Input: part model. Units: mm. Frame: model coordinates. Face numbers are marked on the shaded views. A direction names the side the tool comes from. Round coordinates to 2 decimals unless told otherwise and drop trailing zeros. Loops run counter-clockwise (first coordinate to the right, second up) from the corner with the lowest first, then second, coordinate; pieces in that order, holes last.
1) Section D-D, the plane x = 56.65. Return loops of the section in (y, z).
2) Section B-B, the plane x = 41.15. Return loops of the section in (y, z).
3) Section C-C, the plane z = 12. State how many separate pieces and enclosed holes the cut face has, and give its area (4 significant figures).
4) Access query for the marked faces 5, 6, 7, 8 and 9. Directions: +Z, -Z, +X, -X, +Y, -Y. A direction counts if a zero-diameter tool reaches every point of the face in a straight line with its end or side. Return the directions, or none.
5) Draft query along X for the marked faces 1, 2, 3 and 4. Return one class per face: pulls with the +X half, pulls with the -X half, needs draft (parallel to the pull), parting line crosses it, or undercut.
6) First-contact query: pin 1 (7.5 mm diameter, centred on x = 56.65, y = 14.35, fed in from +Z); pin 2 (4 mm diameter, centred on x = 25.65, y = 44.5, fed in from +Z); pin 3 (4 mm diameter, centred on y = 41, z = 7, fed in from -X); pin 4 (4.5 mm diameter, centred on y = 37, z = 7.5, fed in from +X). Flat tips, straight axial feed; report the tip coordinate or a pass-through.
7) Ray query, line 1 along Y through (x, z) = (56.65, 2.5); line 2 along X through (y, z) = (10, 3.8); line 3 along Y through (x, z) = (56.65, 12.85). Return the intervals inside material, ascending.
8) Section A-A, the plane y = 10. Return loops of the section in (x, z), and give its area (3 significant figures).
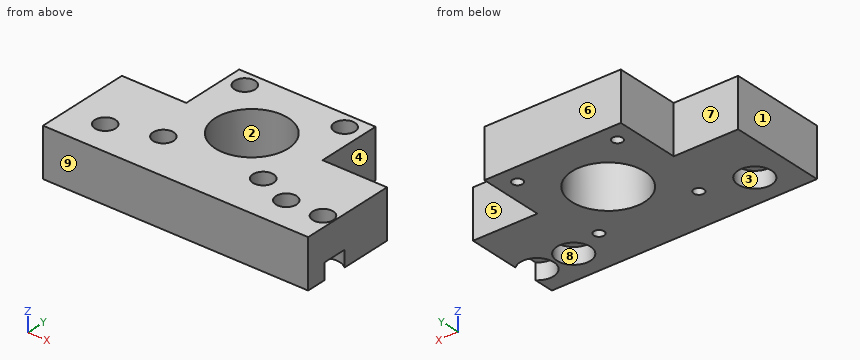
from build123d import *

# Parameters (mm, degrees)
SKETCH_R        = 11.3
SKETCH_R_2      = 1.6
SKETCH_R_3      = 3.2
PAD_DEPTH       = 15
SKETCH001_R     = 3.2
POCKET_DEPTH    = 4
SKETCH002_R     = 5.2
POCKET001_DEPTH = 5


with BuildPart() as part:
    # Sketch → Pad (new body)
    with BuildSketch(Plane.XY):
        Polygon((20, 30), (20, 50.15), (62.3, 50.15), (62.3, 30), (82.3, 30), (82.3, 0), (0, 0), (0, 30), align=None)
        with Locations((41.15, 29)):
            Circle(SKETCH_R, mode=Mode.SUBTRACT)
        with Locations((25.65, 44.5)):
            Circle(SKETCH_R_2, mode=Mode.SUBTRACT)
        with Locations((25.65, 13.5)):
            Circle(SKETCH_R_2, mode=Mode.SUBTRACT)
        with Locations((56.65, 44.5)):
            Circle(SKETCH_R_2, mode=Mode.SUBTRACT)
        with Locations((56.65, 13.5)):
            Circle(SKETCH_R_2, mode=Mode.SUBTRACT)
        with Locations((11.15, 10)):
            Circle(SKETCH_R_3, mode=Mode.SUBTRACT)
        with Locations((67.35, 10)):
            Circle(SKETCH_R_3, mode=Mode.SUBTRACT)
        with Locations((78.75, 10)):
            Circle(SKETCH_R_3, mode=Mode.SUBTRACT)
    extrude(amount=PAD_DEPTH)

    # Sketch001 (on Face18 of Pad) → Pocket (cut)
    with BuildSketch(Plane.XY.offset(15)):
        with Locations((25.65, 45.35)):
            Circle(SKETCH001_R)
        with Locations((56.65, 45.35)):
            Circle(SKETCH001_R)
        with Locations((56.65, 14.35)):
            Circle(SKETCH001_R)
        with Locations((25.65, 14.35)):
            Circle(SKETCH001_R)
    extrude(amount=-POCKET_DEPTH, mode=Mode.SUBTRACT)

    # Sketch002 (on Face4 of Pocket) → Pocket001 (cut)
    with BuildSketch(Plane(origin=(0, 0, 0), x_dir=(1, 0, 0), z_dir=(0, 0, -1))):
        with Locations((11.15, -10)):
            Circle(SKETCH002_R)
        with Locations((67.35, -10)):
            Circle(SKETCH002_R)
        with Locations((78.75, -10)):
            Circle(SKETCH002_R)
    extrude(amount=-POCKET001_DEPTH, mode=Mode.SUBTRACT)


solid = part.part
Final values:
1. outline: (0, 0) - (11.9, 0) - (11.9, 11) - (11.15, 11) - (11.15, 15) - (0, 15) - close; (15.1, 0) - (42.9, 0) - (42.9, 11) - (42.15, 11) - (42.15, 15) - (17.55, 15) - (17.55, 11) - (15.1, 11) - close; (46.1, 0) - (50.15, 0) - (50.15, 15) - (48.55, 15) - (48.55, 11) - (46.1, 11) - close
2. outline: (0, 0) - (17.7, 0) - (17.7, 15) - (0, 15) - close; (40.3, 0) - (50.15, 0) - (50.15, 15) - (40.3, 15) - close
3. separate pieces: 1
3. enclosed holes: 8
3. area: 2,695 mm2
4. face 5: +Z, -Z, +X, +Y
4. face 6: +Z, -Z, +X, -X, +Y
4. face 7: +Z, -Z, -X, +Y
4. face 8: -Z
4. face 9: +Z, -Z, +X, -X, -Y
5. face 1: pulls with the -X half
5. face 2: undercut
5. face 3: undercut
5. face 4: pulls with the +X half
6. pin 1: stops at z = 15
6. pin 2: stops at z = 11
6. pin 3: stops at x = 20
6. pin 4: stops at x = 62.3
7. line 1: y = 0 to 11.9, 15.1 to 42.9, 46.1 to 50.15
7. line 2: x = 0 to 5.95, 16.35 to 62.15, 72.55 to 73.55
7. line 3: y = 0 to 11.15, 17.55 to 42.15, 48.55 to 50.15
8. outline: (0, 0) - (5.95, 0) - (5.95, 5) - (7.95, 5) - (7.95, 15) - (0, 15) - close; (14.35, 5) - (16.35, 5) - (16.35, 0) - (62.15, 0) - (62.15, 5) - (64.15, 5) - (64.15, 15) - (14.35, 15) - close; (70.55, 5) - (72.55, 5) - (72.55, 0) - (73.55, 0) - (73.55, 5) - (75.55, 5) - (75.55, 15) - (70.55, 15) - close; (81.95, 5) - (82.3, 5) - (82.3, 15) - (81.95, 15) - close
8. area: 895 mm2
